from build123d import *

# Parameters (mm, degrees)
F0_R            = 8.3956500105
F0_R_2          = 7.5822661832
F1_DEPTH        = 20
F4_DEPTH        = 25
F5_R            = 3
F6_DEPTH        = 10
F8_R            = 3
F9_DEPTH        = 40
F11_D           = 8.5
F11_DEPTH       = 15
F11_CSINK_D     = 16
F11_CSINK_ANGLE = 90
F11_TIP         = 2.5536576309


with BuildPart() as f1:
    # F0 (on Front) → F1 (new body)
    with BuildSketch(Plane.XZ):
        with BuildLine():
            Line((-17.5, 24.8610879062), (-17.5, -25.1389120938))
            Line((-17.5, -25.1389120938), (17.5, -25.1389120938))
            Line((17.5, -25.1389120938), (17.5, 24.8610879062))
            ThreePointArc((17.5, 24.8610879062), (0, 42.3610879062), (-17.5, 24.8610879062))
        make_face()
        Circle(F0_R, mode=Mode.SUBTRACT)
        with Locations((0, 24.8610879062)):
            Circle(F0_R_2, mode=Mode.SUBTRACT)
    extrude(amount=F1_DEPTH)

    # F3 (on face) → F4 (cut)
    with BuildSketch(Plane.XZ.offset(20)):
        Polygon((-10, -19.1389120938), (-6.0486232505, -24.7820629224), (8.8115125525, -19.1389120938), align=None)
        Polygon((-6.0486232505, -24.7820629224), (-5.7255781316, -25.2434191651), (5.7496010901, -25.2091108247), (8.3105433405, -21.5517062546), (8.9213285707, -19.1389120938), (8.8115125525, -19.1389120938), align=None)
        Polygon((8.9213285707, -19.1389120938), (8.3105433405, -21.5517062546), (10, -19.1389120938), align=None)
    extrude(amount=-F4_DEPTH, mode=Mode.SUBTRACT)

    # F5 (on face) → F6 (cut)
    with BuildSketch(Plane.YZ.offset(17.5)):
        with Locations((-10, 0)):
            Circle(F5_R)
    extrude(amount=-F6_DEPTH, mode=Mode.SUBTRACT)

    # F8 (on offset) → F9 (cut)
    with BuildSketch(Plane.XY.offset(67.5)):
        with Locations((0, -10)):
            Circle(F8_R)
    extrude(amount=-F9_DEPTH, mode=Mode.SUBTRACT)

    # F11
    with Locations(Plane(origin=(0, 0, 0), x_dir=(-1, 0, 0), z_dir=(0, 1, 0))):
        with Locations((10, 13), (-10.7969033529, 13)):
            CounterSinkHole(F11_D / 2, F11_CSINK_D / 2, depth=F11_DEPTH, counter_sink_angle=F11_CSINK_ANGLE)
            with Locations((0, 0, -(F11_DEPTH + F11_TIP / 2))):  # 118° drill point
                Cone(0, F11_D / 2, F11_TIP, mode=Mode.SUBTRACT)


solid = f1.part
Verification items for the finished model (mm, model axes). A direction names the side the tool comes from. Give positions to 0.01 mm unless a question says otherwise; leave off trailing zeros. Loops run counter-clockwise (first coordinate to the right, second up) from the corner with the lowest first, then second, coordinate; pieces in that order, holes last.
1. Cross-section at A-A on z = 0. Record the cut outline in (x, y).
Derived:
outline: (-17.5, -20) - (-8.4, -20) - (-8.4, 0) - (-17.5, 0) - close; (8.4, -20) - (17.5, -20) - (17.5, -13) - (8.4, -13) - close; (8.4, -7) - (17.5, -7) - (17.5, 0) - (8.4, 0) - close
2. Material ranges on probe 1 along X at (y, z) = (-12.25, 13); probe 2 along Z at (x, y) = (0, -15); probe 3 along Z at (x, y) = (0, -12), recorded low to high.
Derived:
probe 1: x = -17.5 to -14.25, -5.75 to 6.55, 15.05 to 17.5
probe 2: z = -19.14 to -8.4, 8.4 to 17.28, 32.44 to 42.36
probe 3: z = -19.14 to -8.4, 8.4 to 17.28
3. Cross-section at D-D on y = -3. Record the cut outline in (x, z).
Derived:
outline: (-17.5, -25.14) - (-5.8, -25.14) - (-10, -19.14) - (10, -19.14) - (5.8, -25.14) - (17.5, -25.14) - (17.5, 24.86) arc R17.5 ccw to (-17.5, 24.86) - close; hole circle Ø10 at (-10, 13); hole circle Ø16.79 at (0, 0); hole circle Ø15.16 at (0, 24.86); hole circle Ø10 at (10.8, 13)
4. Go/stop test with flat-tipped pins: P1, Ø12, axis at x = 0, z = 24.86, coming from the -Y side; P2, Ø3, axis at x = -12, y = -5.5, coming from the +Z side; P3, Ø3.5, axis at x = 0, y = -10, coming from the +Z side; P4, Ø2, axis at y = -3.5, z = 28.5, coming from the +X side. Record where each tip stops, or that it passes through.
Derived:
P1: passes through
P2: stops at z = 38.86
P3: stops at z = 17.48
P4: stops at x = 17.3
5. Release check for a two-part mould opening along X. For faces 1 (the cylindrical face through (0.385, -5.416, 42.357)), 2 (the flat face through (0, 0, 9)), 3 (the cylindrical face through (-10.92, -9.45, 8.85)) record: +X half, -X half, draft (parallel to the pull), parting line (faces both ways), or undercut.
Derived:
face 1: parting line
face 2: draft
face 3: undercut
6. Tool access check on faces 4 (the cylindrical face through (0, -7, 37)), 5 (the cylindrical face through (14.72, -9.45, 11.37)), 6 (the flat face through (0, -10, -19.139)), 7 (the cylindrical face through (12.7, -12.4, -1.8)). Record the directions out of +Z, -Z, +X, -X, +Y, -Y that give a thin tool (end or side, any length) a straight path to the whole face; none if there is none.
Derived:
face 4: +Z
face 5: +Y
face 6: +Y, -Y
face 7: +X
7. Cross-section at C-C on y = -12. Record the cut outline in (x, z).
Derived:
outline: (-17.5, -25.14) - (-5.8, -25.14) - (-10, -19.14) - (10, -19.14) - (5.8, -25.14) - (17.5, -25.14) - (17.5, -2.24) - (8.09, -2.24) arc R8.4 cw (long way) to (8.09, 2.24) - (17.5, 2.24) - (17.5, 24.86) arc R17.5 ccw to (2.24, 42.22) - (2.24, 32.11) arc R7.58 cw (long way) to (-2.24, 32.11) - (-2.24, 42.22) arc R17.5 ccw to (-17.5, 24.86) - close; hole circle Ø8.5 at (-10, 13); hole circle Ø8.5 at (10.8, 13)
8. Cross-section at B-B on x = 0. Record the cut outline in (y, z).
Derived:
outline: (-20, -19.14) - (0, -19.14) - (0, -8.4) - (-20, -8.4) - close; (-20, 8.4) - (0, 8.4) - (0, 17.28) - (-20, 17.28) - close; (-20, 32.44) - (-13, 32.44) - (-13, 42.36) - (-20, 42.36) - close; (-7, 32.44) - (0, 32.44) - (0, 42.36) - (-7, 42.36) - close
